Geometry check sheet. Reference: drawing and pictorial views, mm from the part's lowest x, y, z. Round coordinates to 2 decimals unless told otherwise and drop trailing zeros. Loops run counter-clockwise (first coordinate to the right, second up) from the corner with the lowest first, then second, coordinate; pieces in that order, holes last. Notation, with made-up numbers: (-20, -23) - (12, -23) arc R32 cw to (12, 7) - close; hole circle Ø3 at (-3, 63). An arc over 180 degrees is marked (long way). Return JSON: item names as keys, results as strings.
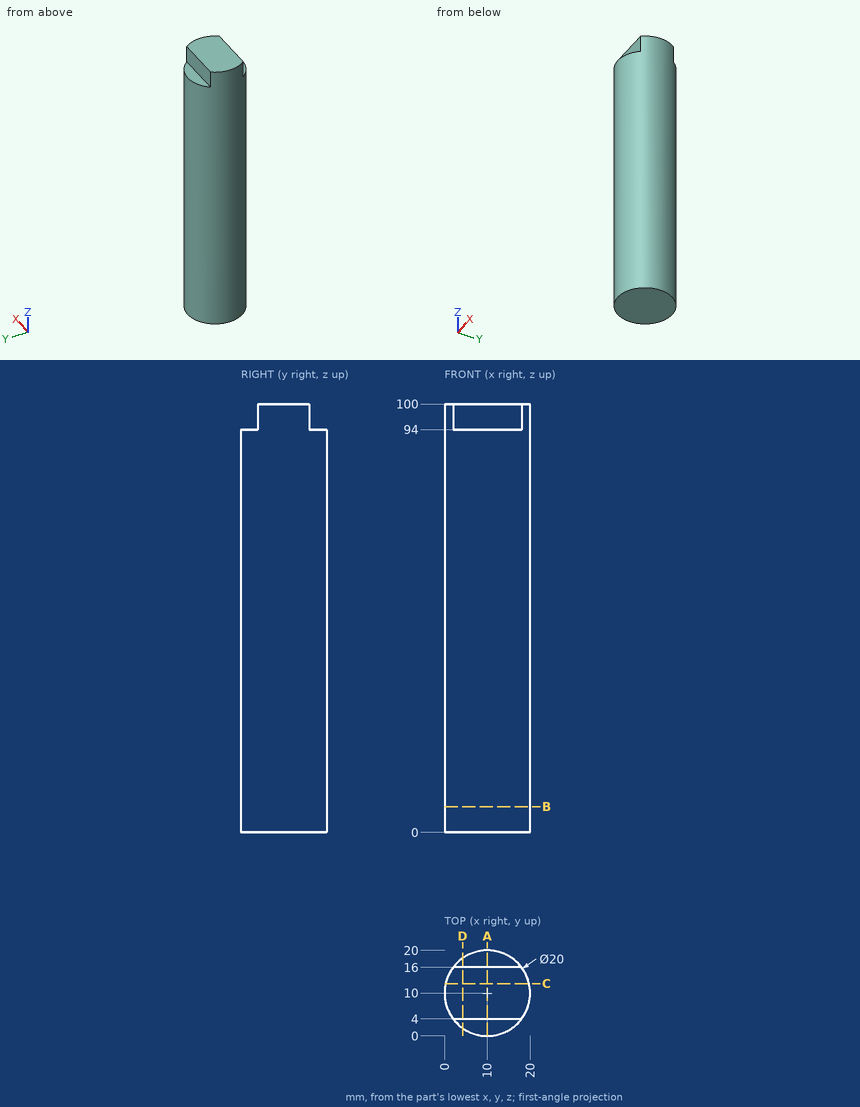
Q1. Depth check by flat-ended pin: P1, Ø2, axis at x = 8, y = 18, coming from the +Z side; P2, Ø3, axis at x = 4.5, z = 55.5, coming from the -Y side; P3, Ø3, axis at x = 12.5, z = 97.5, coming from the -Y side. Enter the tip coordinate at first touch or a pass-through.
Answer key:
{"P1": "stops at z = 94", "P2": "stops at y = 0.83", "P3": "stops at y = 4"}
Q2. Sectioned sample at B-B (z = 6). Enter the section's corners in (x, y).
Answer key:
{"outline": "circle Ø20 at (10, 10)"}
Q3. Sectioned sample at D-D (x = 4.25). Enter the section's corners in (y, z).
Answer key:
{"outline": "(1.82, 0) - (18.18, 0) - (18.18, 94) - (16, 94) - (16, 100) - (4, 100) - (4, 94) - (1.82, 94) - close"}
Q4. Scan lines: probe 1 along X at (y, z) = (16, 78); probe 2 along Z at (x, y) = (6, 2). Record each from-to range of solid material in increasing order. Write a range as [from, to].
Answer key:
{"probe 1": "x = [2, 18]", "probe 2": "z = [0, 94]"}
Q5. Sectioned sample at C-C (y = 12.25). Enter the section's corners in (x, z).
Answer key:
{"outline": "(0.26, 0) - (19.74, 0) - (19.74, 100) - (0.26, 100) - close"}
Q6. Sectioned sample at A-A (x = 10). Enter the section's corners in (y, z), plus the area to 3 significant figures.
Answer key:
{"outline": "(0, 0) - (20, 0) - (20, 94) - (16, 94) - (16, 100) - (4, 100) - (4, 94) - (0, 94) - close", "area": "1,950 mm²"}
